Design review of the part shown in the three views and the two pictorial views. Dimensions are in mm from the part's minimum x, y and z. A direction names the side the tool comes from. Round coordinates to 2 decimals unless told otherwise and drop trailing zeros. Loops run counter-clockwise (first coordinate to the right, second up) from the corner with the lowest first, then second, coordinate; pieces in that order, holes last. Notation, with made-up numbers: (55.5, 81.5) - (111.5, 81.5) arc R28 cw to (111.5, 104.5) - close; hole circle Ø8 at (-24, 44.5). An arc over 180 degrees is marked (long way). Return JSON: item names as keys, results as strings. Group by question number.
(1) The part is to be moulded in two halves that separate along Y. For the marked faces 1, 2 and 3, say which applies: pulls with the +Y half, pulls with the -Y half, needs draft (parallel to the pull), parting line crosses it, or undercut.
(2) We need section B-B, the plane x = 27.5. Write out the cut boundary in (y, z).
(3) Wall thickness on L1, parallel to Y at x = 27.5, z = 10; L2, parallel to Z at x = 7.5, y = 15; L3, parallel to X at y = 15.5, z = 6 (1 decimal): over which ranges is each line inside the solid? List them lowest first. Write a range as [from, to].
(4) We need section A-A, the plane y = 15. Write out the cut boundary in (x, z), and give its area (3 significant figures).
(5) For the marked faces 4 and 5, list the 3-axis set-ups (+Z, -Z, +X, -X, +Y, -Y) from which the entire face can be reached by the end or side of a thin tool; tool diameter is ignored.
(6) We need section C-C, the plane z = 3. Write out the cut boundary in (x, y).
(7) We need section D-D, the plane y = 24.25. Write out the cut boundary in (x, z).
(8) Clearance check with a flat-ended pin moving along its axis: pin 1 (9 mm diameter, centred on x = 27.5, y = 15, fed in from -Z). State where the tip first meets the part, or that it passes through.
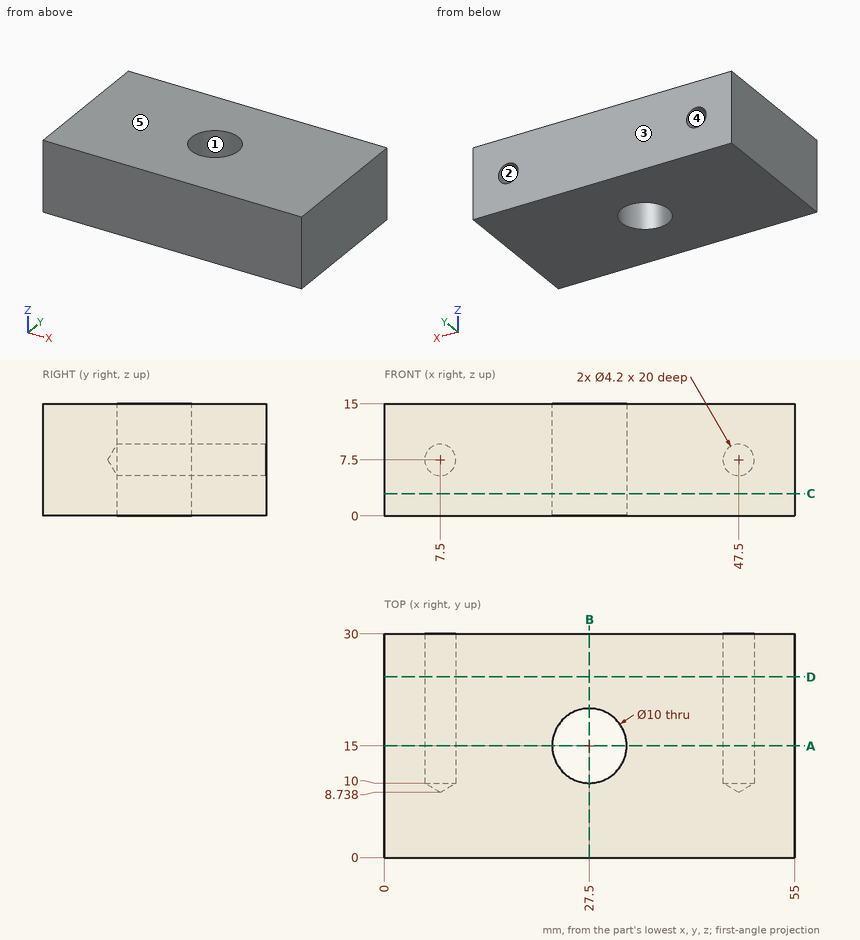
Solutions:
{
 "1": {"face 1": "undercut", "face 2": "needs draft", "face 3": "pulls with the +Y half"},
 "2": {"outline": "(0, 0) - (10, 0) - (10, 15) - (0, 15) - close; (20, 0) - (30, 0) - (30, 15) - (20, 15) - close"},
 "3": {"L1": "[0, 10], [20, 30]", "L2": "[0, 5.4], [9.6, 15]", "L3": "[0, 6], [9, 22.5], [32.5, 46], [49, 55]"},
 "4": {"outline": "(0, 0) - (22.5, 0) - (22.5, 15) - (0, 15) - close; (32.5, 0) - (55, 0) - (55, 15) - (32.5, 15) - close; hole circle Ø4.2 at (7.5, 7.5); hole circle Ø4.2 at (47.5, 7.5)", "area": "647 mm^2"},
 "5": {"face 4": "+Y", "face 5": "+Z, +X, -X, +Y, -Y"},
 "6": {"outline": "(0, 0) - (55, 0) - (55, 30) - (0, 30) - close; hole circle Ø10 at (27.5, 15)"},
 "7": {"outline": "(0, 0) - (55, 0) - (55, 15) - (0, 15) - close; hole circle Ø4.2 at (7.5, 7.5); hole circle Ø4.2 at (47.5, 7.5)"},
 "8": {"pin 1": "through"}
}
